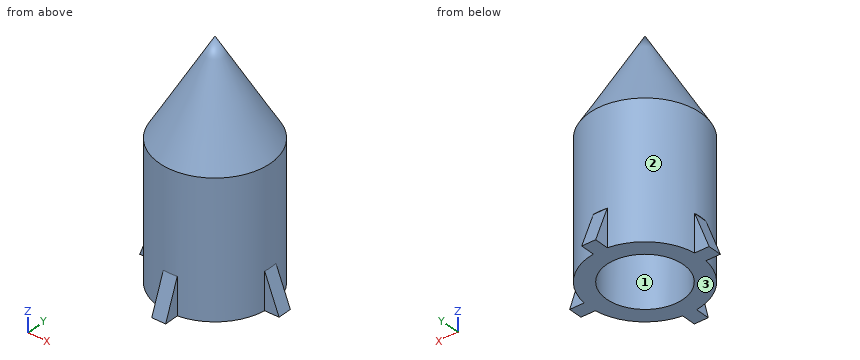
```python
from build123d import *

# Parameters (mm, degrees)
F0_W      = 76.2
F0_H      = 184.446418
F2_R      = 52.454734
F3_DEPTH  = 76.2
F4_W      = 38.1
F4_H      = 9.525
F4_W_2    = 9.525
F4_H_2    = 38.1
F5_DEPTH  = 50.8
F7_DEPTH  = 104.776
F9_DEPTH  = 104.776
F11_DEPTH = 104.776
F13_DEPTH = 104.776


with BuildPart() as f1:
    # F0 (on Right) → F1 (revolve)
    with BuildSketch(Plane.YZ):
        Polygon((-76.2, 92.223209), (0, 92.223209), (0, 223.083655), align=None)
        with Locations((-38.1, 0)):
            Rectangle(F0_W, F0_H)
    revolve(axis=Axis((0, 0, 0), (0, 0, -1)))

    # F2 (on face) → F3 (cut)
    with BuildSketch(Plane(origin=(0, 0, -92.223209), x_dir=(1, 0, 0), z_dir=(0, 0, -1))):
        Circle(F2_R)
    extrude(amount=-F3_DEPTH, mode=Mode.SUBTRACT)

    # F4 (on face) → F5 (join)
    with BuildSketch(Plane(origin=(0, 0, -92.223209), x_dir=(1, 0, 0), z_dir=(0, 0, -1))):
        with Locations((76.2, -4.7625)):
            Rectangle(F4_W, F4_H)
        with Locations((76.2, 4.7625)):
            Rectangle(F4_W, F4_H)
        with Locations((-76.2, -4.7625)):
            Rectangle(F4_W, F4_H)
        with Locations((4.7625, 76.2)):
            Rectangle(F4_W_2, F4_H_2)
        with Locations((-4.7625, 76.2)):
            Rectangle(F4_W_2, F4_H_2)
        with Locations((-76.2, 4.7625)):
            Rectangle(F4_W, F4_H)
        Polygon((9.525, -57.15), (0, -57.15), (-9.525, -57.15), (-9.525, -95.25), (9.525, -95.25), align=None)
    extrude(amount=-F5_DEPTH)

    # F6 (on face) → F7 (cut, through all)
    with BuildSketch(Plane.XZ.offset(9.525)):
        Polygon((-95.25, -41.423209), (-95.25, -92.223209), (-75.602344, -41.423209), align=None)
    extrude(amount=-F7_DEPTH, mode=Mode.SUBTRACT)

    # F8 (on face) → F9 (cut, through all)
    with BuildSketch(Plane.YZ.offset(9.525)):
        Polygon((-95.25, -41.423209), (-95.25, -92.223209), (-75.602344, -41.423209), (-85.426172, -41.423209), align=None)
    extrude(amount=-F9_DEPTH, mode=Mode.SUBTRACT)

    # F10 (on face) → F11 (cut, through all)
    with BuildSketch(Plane(origin=(-9.525, 0, 0), x_dir=(0, -1, 0), z_dir=(-1, 0, 0))):
        Polygon((-95.25, -41.423209), (-95.25, -92.223209), (-75.602344, -41.423209), align=None)
    extrude(amount=-F11_DEPTH, mode=Mode.SUBTRACT)

    # F12 (on face) → F13 (cut, through all)
    with BuildSketch(Plane(origin=(0, 9.525, 0), x_dir=(-1, 0, 0), z_dir=(0, 1, 0))):
        Polygon((-95.25, -41.423209), (-95.25, -92.223209), (-75.602344, -41.423209), align=None)
    extrude(amount=-F13_DEPTH, mode=Mode.SUBTRACT)


solid = f1.part
```
Build history of the part. All positions in model axes, mm. Face numbers are marked on the shaded views. Round coordinates to 2 decimals unless told otherwise and drop trailing zeros. Write each loop counter-clockwise with the first axis right and the second up, starting at its lowest first coordinate (ties: lowest second). Pieces come first, ordered by that corner, then holes.
1) Band-saw the part on C-C, the plane y = 80.5. List the corners of the cut face in (x, z) (3 decimals), and give its area (3 significant figures).
2) Drill centre lines: probe 1 along X at (y, z) = (0, -38); probe 2 along X at (y, z) = (0, -50); probe 3 along Y at (x, z) = (0, -57). Where is each one in solid material? Low to high.
3) Band-saw the part on A-A, the plane z = -49. List the corners of the cut face in (x, y) (3 decimals).
4) Band-saw the part on B-B, the plane z = 14. List the corners of the cut face in (x, y).
5) Pin check, flat tips, straight feed: pin 1 (10 mm diameter, centred on y = -87, z = -66, fed in from +X) (3 decimals); pin 2 (6 mm diameter, centred on x = 34, y = 52.5, fed in from +Z); pin 3 (6 mm diameter, centred on y = 89.5, z = -64.5, fed in from +X); pin 4 (8 mm diameter, centred on x = 39.5, y = -24, fed in from -Z). Stop position of each tip, or through.
6) Mould opens along Y. For the marked faces 1, 2 and 3 say: +Y half, -Y half, draft (parallel to the pull), parting line (faces both ways), or undercut.
7) Band-saw the part on D-D, the plane z = 194. List the corners of the cut face in (x, y).
Ans:
1. outline: (-9.525, -92.223) - (9.525, -92.223) - (9.525, -54.086) - (-9.525, -54.086) - close
1. area: 727 mm2
2. probe 1: x = -76.2 to -52.45, 52.45 to 76.2
2. probe 2: x = -78.92 to -52.45, 52.45 to 78.92
2. probe 3: y = -81.63 to -52.45, 52.45 to 81.63
3. outline: (-78.533, -9.525) - (-75.602, -9.525) arc R76.2 ccw to (-9.525, -75.602) - (-9.525, -78.533) - (9.525, -78.533) - (9.525, -75.602) arc R76.2 ccw to (75.602, -9.525) - (78.533, -9.525) - (78.533, 9.525) - (75.602, 9.525) arc R76.2 ccw to (9.525, 75.602) - (9.525, 78.533) - (-9.525, 78.533) - (-9.525, 75.602) arc R76.2 ccw to (-75.602, 9.525) - (-78.533, 9.525) - close; hole circle Ø104.909 at (0, 0)
4. outline: circle Ø152.4 at (0, 0)
5. pin 1: stops at x = 9.525
5. pin 2: stops at z = 120.82
5. pin 3: passes through
5. pin 4: stops at z = -16.02
6. face 1: undercut
6. face 2: parting line
6. face 3: draft
7. outline: circle Ø33.87 at (0, 0)
